Geometry: final body of the model. Coordinates: model frame, mm. A direction names the side the tool comes from. Give positions to 0.01 mm unless a question says otherwise; leave off trailing zeros. Write each loop counter-clockwise with the first axis right and the second up, starting at its lowest first coordinate (ties: lowest second). Pieces come first, ordered by that corner, then holes.
Q1. Cut plane D-D on z = -22. Return the cut outline in (x, y).
Q2. Cut plane C-C on z = -3.5. Return the cut outline in (x, y).
Q3. Cut plane B-B on y = 10. Return the cut outline in (x, z) (3 decimals), plus the area to 3 significant figures.
Q4. Cut plane A-A on x = 0. Return the cut outline in (y, z) (3 decimals), plus the area to 3 significant figures.
Q5. Draft query along X for faces 1 (the face through (0, 25.4, -12)), 2 (the face through (53.74, -7.76, 23.64)), 3 (the face through (14, 0, 0)). Return one class per face: pulls with the +X half, pulls with the -X half, needs draft (parallel to the pull), parting line crosses it, or undercut.
Q6. Pin query (flat end, axial travel): pin 1 (8.5 mm diameter, centred on x = 14, y = 16.5, fed in from +Z); pin 2 (8.5 mm diameter, centred on x = -15, y = 5.5, fed in from +Z); pin 3 (1 mm diameter, centred on y = 6.5, z = -3.5, fed in from -X); pin 4 (6 mm diameter, centred on x = 15.5, z = 0, fed in from +Y). Return the tip coordinate at first contact, or that it passes through.
Q7. Line query: L1, parallel to Y at x = 90, z = -9; L2, parallel to X at y = 16, z = -4; L3, parallel to X at y = -13.5, z = 7.5. Output: solid intervals per line, ascending.
Q8. Reachability of faces 4 (the face through (-17.78, 5, 0)), 5 (the face through (14, 13, -5.08)), 6 (the face through (45, -15.748, 0)) from +Z, -Z, +X, -X, +Y, -Y: full face, straight path, thin tool, end or side. Return the list, or none.
```python
from build123d import *
from build123d import SkipClean  # not in build123d's __all__

# Parameters (mm, degrees)
F0_R     = 11.43
F1_DEPTH = 15.748
F2_DEPTH = 25.4


with BuildPart() as f1:
    # F0 (on Front) → F1 (new body)
    with BuildSketch(Plane.XZ):
        with BuildLine():
            ThreePointArc((2.67890625, 28.4491491315), (21.1314974753, 19.2351355455), (28.575, 0))
            ThreePointArc((28.575, 0), (21.1314974753, -19.2351355455), (2.67890625, -28.4491491315))
            Line((2.67890625, -28.4491491315), (103.3859375, -18.966099421))
            ThreePointArc((103.3859375, -18.966099421), (82.55, 0), (103.3859375, 18.966099421))
            Line((103.3859375, 18.966099421), (2.67890625, 28.4491491315))
        make_face()
        with BuildLine():
            ThreePointArc((2.67890625, -28.4491491315), (21.1314974753, -19.2351355455), (28.575, 0))
            ThreePointArc((28.575, 0), (21.1314974753, 19.2351355455), (2.67890625, 28.4491491315))
            ThreePointArc((2.67890625, 28.4491491315), (-28.575, 0), (2.67890625, -28.4491491315))
        make_face()
        with BuildLine():
            ThreePointArc((-10.2390673403, 5.08), (0, 11.43), (10.2390673403, 5.08))
            Line((10.2390673403, 5.08), (17.78, 5.08))
            Line((17.78, 5.08), (17.78, -5.08))
            Line((17.78, -5.08), (10.2390673403, -5.08))
            ThreePointArc((10.2390673403, -5.08), (0, -11.43), (-10.2390673403, -5.08))
            Line((-10.2390673403, -5.08), (-17.78, -5.08))
            Line((-17.78, -5.08), (-17.78, 5.08))
            Line((-17.78, 5.08), (-10.2390673403, 5.08))
        make_face(mode=Mode.SUBTRACT)
        with BuildLine():
            ThreePointArc((120.65, 0), (115.6876649835, 12.823423697), (103.3859375, 18.966099421))
            ThreePointArc((103.3859375, 18.966099421), (82.55, 0), (103.3859375, -18.966099421))
            ThreePointArc((103.3859375, -18.966099421), (115.6876649835, -12.823423697), (120.65, 0))
        make_face()
        with Locations((101.6, 0)):
            Circle(F0_R, mode=Mode.SUBTRACT)
        with Locations((101.6, 0)):
            Circle(F0_R)
        with BuildLine():
            ThreePointArc((10.2390673403, 5.08), (11.1282846769, 2.6088656826), (11.43, 0))
            ThreePointArc((11.43, 0), (11.1282846769, -2.6088656826), (10.2390673403, -5.08))
            Line((10.2390673403, -5.08), (17.78, -5.08))
            Line((17.78, -5.08), (17.78, 5.08))
            Line((17.78, 5.08), (10.2390673403, 5.08))
        make_face()
    extrude(amount=F1_DEPTH)

    # F0 (on Front) → F2 (join)
    with BuildSketch(Plane.XZ):
        with BuildLine():
            ThreePointArc((2.67890625, -28.4491491315), (21.1314974753, -19.2351355455), (28.575, 0))
            ThreePointArc((28.575, 0), (21.1314974753, 19.2351355455), (2.67890625, 28.4491491315))
            ThreePointArc((2.67890625, 28.4491491315), (-28.575, 0), (2.67890625, -28.4491491315))
        make_face()
        with BuildLine():
            ThreePointArc((-10.2390673403, 5.08), (0, 11.43), (10.2390673403, 5.08))
            Line((10.2390673403, 5.08), (17.78, 5.08))
            Line((17.78, 5.08), (17.78, -5.08))
            Line((17.78, -5.08), (10.2390673403, -5.08))
            ThreePointArc((10.2390673403, -5.08), (0, -11.43), (-10.2390673403, -5.08))
            Line((-10.2390673403, -5.08), (-17.78, -5.08))
            Line((-17.78, -5.08), (-17.78, 5.08))
            Line((-17.78, 5.08), (-10.2390673403, 5.08))
        make_face(mode=Mode.SUBTRACT)
    with SkipClean():  # cleaning this boolean's faces spoils the solid; the shape is the same uncleaned
        extrude(amount=-F2_DEPTH)


solid = f1.part
```
Data:
1. outline: (-18.24, -15.75) - (71.17, -15.75) - (71.17, 0) - (18.24, 0) - (18.24, 25.4) - (-18.24, 25.4) - close
2. outline: (-28.36, -15.75) - (-17.78, -15.75) - (-17.78, 25.4) - (-28.36, 25.4) - close; (10.88, -15.75) - (120.33, -15.75) - (120.33, 0) - (28.36, 0) - (28.36, 25.4) - (17.78, 25.4) - (17.78, 0) - (10.88, 0) - close
3. outline: circle Ø57.15 at (0, 0); hole (-17.78, -5.08) - (-10.239, -5.08) arc R11.43 ccw to (10.239, -5.08) - (17.78, -5.08) - (17.78, 5.08) - (10.239, 5.08) arc R11.43 ccw to (-10.239, 5.08) - (-17.78, 5.08) - close
3. area: 2,020 mm2
4. outline: (-15.748, -28.575) - (25.4, -28.575) - (25.4, -11.43) - (-15.748, -11.43) - close; (-15.748, 11.43) - (25.4, 11.43) - (25.4, 28.575) - (-15.748, 28.575) - close
4. area: 1,410 mm2
5. face 1: needs draft
5. face 2: pulls with the +X half
5. face 3: undercut
6. pin 1: stops at z = 26.86
6. pin 2: stops at z = 26.48
6. pin 3: stops at x = -28.42
6. pin 4: stops at y = 25.4
7. L1: y = -15.75 to 0
7. L2: x = -28.29 to -17.78, 17.78 to 28.29
7. L3: x = -27.57 to -8.63, 8.63 to 119.11
8. face 4: +Y, -Y
8. face 5: +Y
8. face 6: +Z, -Z, +X, -X, -Y
